```python
from build123d import *

# Parameters (mm, degrees)
SKETCH1_R           = 22.5
SKETCH1_R_2         = 21
BOSS_EXTRUDE1_DEPTH = 34.5


with BuildPart() as part:
    # Sketch1 → Boss-Extrude1 (new body)
    with BuildSketch(Plane(origin=(0, 0, 0), x_dir=(1, 0, 0), z_dir=(0, 1, 0))):
        with Locations(Location((0, 0, 0), (0, 0, 270))):
            Circle(SKETCH1_R)
        with Locations(Location((0, 0, 0), (0, 0, 270))):
            Circle(SKETCH1_R_2, mode=Mode.SUBTRACT)
    extrude(amount=BOSS_EXTRUDE1_DEPTH)

    # Sketch5 → Revolve1 (revolve)
    with BuildSketch(Plane.XY, mode=Mode.PRIVATE) as revolve1_sk:
        Polygon((22.5, 34.5), (12, 49.120191517), (12, 59.120191517), (3.5, 59.120191517), (3.5, 49.120191517), (21, 34.5), align=None)
    revolve(revolve1_sk.sketch.rotate(Axis((0, 0, 0), (0, 1, 0)), 90), axis=Axis((0, 0, 0), (0, 1, 0)))

    # Sketch10 → Revolve3 (revolve)
    with BuildSketch(Plane(origin=(0, 0, 0), x_dir=(-1, 0, 0), z_dir=(0, 0, -1)), mode=Mode.PRIVATE) as revolve3_sk:
        Polygon((-3.5, 59.120191517), (-10.526661033, 89.120191517), (-12.026661033, 89.120191517), (-8.25, 59.120191517), align=None)
    revolve(revolve3_sk.sketch.rotate(Axis((0, 59.120191517, 0), (0, 1, 0)), 90), axis=Axis((0, 59.120191517, 0), (0, 1, 0)))


solid = part.part
```
Geometry check sheet. Reference: the model listing, model coordinates, mm. A direction names the side the tool comes from. Coordinates: 2 decimals unless noted, no trailing zeros. Write each loop counter-clockwise with the first axis right and the second up, starting at its lowest first coordinate (ties: lowest second). Pieces come first, ordered by that corner, then holes. Notation, with made-up numbers: (55.25, 87) -> (63.25, 87) arc R18 cw to (63.25, 105) -> close; hole circle Ø9 at (42, 36). An arc over 180 degrees is marked (long way). Use CSV: the item, a comma, the result in double quotes. Start each with the question number.
Item 1: Cross-section at A-A, the plane z = 0. Record the cut outline in (x, y), plus the area to 3 significant figures.
Item 2: Cross-section at D-D, the plane y = 69.5. Record the cut outline in (x, z), plus the area to 3 significant figures.
Item 3: Cross-section at C-C, the plane y = 50.5. Record the cut outline in (x, z), plus the area to 3 significant figures.
Item 4: Thickness scan on line 1 (X direction, y = 56, z = 0); line 2 (X direction, y = 12, z = 5.5); line 3 (Z direction, x = 9, y = 12). Record the ranges inside material, lowest first.
Item 5: Cross-section at B-B, the plane x = 0. Record the cut outline in (y, z), plus the area to 3 significant figures.
Item 6: Depth check by flat-ended pin: pin 1 Ø12 at (y, z) = (73, -3) entering from -X; pin 2 Ø10 at (x, z) = (-10.5, -16) entering from -Y; pin 3 Ø1 at (y, z) = (40, -2) entering from +X; pin 4 Ø1 at (x, z) = (-4.5, -1) entering from -Y. Enter the tip coordinate at first touch or a pass-through.
Item 7: Mould release check, pull along X, two halves, no side actions. Record for faces 1 (the conical face through (-1.38, 48.21, -4.38)), 2 (the cylindrical face through (-8.618, 17.008, 20.784)), 3 (the flat face through (11, 89.12, 0)): released by +X, released by -X, zero draft, split by the parting line, or undercut.
Item 8: Set-up check for faces 4 (the flat face through (-20, 0, -7)), 5 (the cylindrical face through (6.31, 17.01, 20.03)), 6 (the cylindrical face through (3.105, 54.05, -1.615)), 7 (the flat face through (8, 59.12, 3)): record each of +Z, -Z, +X, -X, +Y, -Y from which the full face is reachable in a straight line by a thin tool's end or side.
Answers:
1,outline,"(-22.5, 0) -> (-21, 0) -> (-21, 34.5) -> (-3.5, 49.12) -> (-3.5, 59.12) -> (-10.53, 89.12) -> (-12.03, 89.12) -> (-8.25, 59.12) -> (-12, 59.12) -> (-12, 49.12) -> (-22.5, 34.5) -> close; (3.5, 49.12) -> (21, 34.5) -> (21, 0) -> (22.5, 0) -> (22.5, 34.5) -> (12, 49.12) -> (12, 59.12) -> (8.25, 59.12) -> (12.03, 89.12) -> (10.53, 89.12) -> (3.5, 59.12) -> close"
1,area,"607 mm^2"
2,outline,"circle Ø19.11 at (0, 0); hole circle Ø11.86 at (0, 0)"
2,area,"176 mm^2"
3,outline,"circle Ø24 at (0, 0); hole circle Ø7 at (0, 0)"
3,area,"414 mm^2"
4,line 1,"-12 to -3.5, 3.5 to 12"
4,line 2,"-21.82 to -20.27, 20.27 to 21.82"
4,line 3,"-20.62 to -18.97, 18.97 to 20.62"
5,outline,"(0, -22.5) -> (34.5, -22.5) -> (49.12, -12) -> (59.12, -12) -> (59.12, -8.25) -> (89.12, -12.03) -> (89.12, -10.53) -> (59.12, -3.5) -> (49.12, -3.5) -> (34.5, -21) -> (0, -21) -> close; (0, 21) -> (34.5, 21) -> (49.12, 3.5) -> (59.12, 3.5) -> (89.12, 10.53) -> (89.12, 12.03) -> (59.12, 8.25) -> (59.12, 12) -> (49.12, 12) -> (34.5, 22.5) -> (0, 22.5) -> close"
5,area,"607 mm^2"
6,pin 1,"x = -10.67"
6,pin 2,"y = 0"
6,pin 3,"x = 18.81"
6,pin 4,"y = 47.78"
7,face 1,"undercut"
7,face 2,"split by the parting line"
7,face 3,"zero draft"
8,face 4,"+Z, -Z, +X, -X, -Y"
8,face 5,"-Y"
8,face 6,"+Y, -Y"
8,face 7,"none"
